Study the drawing (mm; zero at the part's minimum x, y, z) and answer. A direction names the side the tool comes from. Coordinates: 2 decimals unless noted, no trailing zeros. Write each loop counter-clockwise with the first axis right and the second up, starting at its lowest first coordinate (ties: lowest second). Pieces come first, ordered by that corner, then holes. Notation, with made-up numbers: M -14.75,-29.5 L -6.75,-29.5 A19 cw -6.75,1.5 Z; hole C 59,31 d8. An arc over 180 degrees is marked long. Answer as CSV lines item,"result". Start each with the question number.
(1) A cutting plane is placed at B-B on x = 3. Give the vertices of the cut face in (y, z).
(2) A cutting plane is placed at D-D on z = 0.5. Give the vertices of the cut face in (x, y).
(3) Find the intervals of material crossed by L1, parallel to Z at x = 3, y = 0.8; L2, parallel to X at y = 0.5, z = 4; L3, parallel to Y at x = 2.5, z = 0.85, in increasing order. Write a range as [from, to].
(4) For the marked faces 5, 6 and 7, determine the directions among +Z, -Z, +X, -X, +Y, -Y from which every point of the face is accessible in a straight line to the end or side of a thin tool.
(5) Flat-ended cylindrical pins translate along their axes: P1, Ø1.8, axis at x = 3, z = 2.5, coming from the +Y side; P2, Ø2, axis at x = 18, z = 5, coming from the -Y side. Find the tip coordinate at first contact, or state that the pin passes through.
(6) The mould has two halves that part along X. Classify the marked faces 1, 2, 3 and 4: released by +X, released by -X, zero draft, split by the parting line, or undercut.
(7) A cutting plane is placed at C-C on y = 4.5. Give the vertices of the cut face in (x, z), then the cut area to 3 significant figures.
(8) A cutting plane is placed at A-A on z = 4.2. Give the vertices of the cut face in (x, y), then the cut area to 3 significant figures.
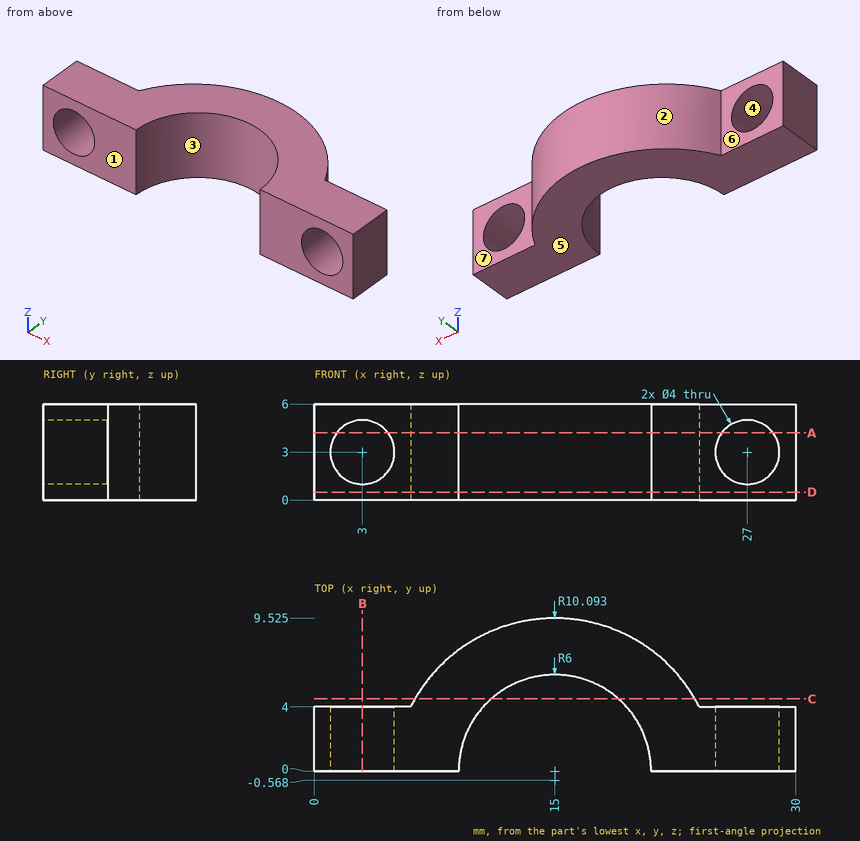
Here are the results:
1,outline,"M 0,0 L 4,0 L 4,1 L 0,1 Z; M 0,5 L 4,5 L 4,6 L 0,6 Z"
2,outline,"M 0,0 L 9,0 A6 cw 21,0 L 30,0 L 30,4 L 24,4 A10.09 ccw 6,4 L 0,4 Z"
3,L1,"z = [0, 1], [5, 6]"
3,L2,"x = [0, 1.27], [4.73, 9.02], [20.98, 25.27], [28.73, 30]"
3,L3,"y = [0, 4]"
4,face 5,"-Z, +X, -X, +Y, -Y"
4,face 6,"+Z, -Z, -X, +Y"
4,face 7,"+Z, -Z, +X, +Y"
5,P1,"passes through"
5,P2,"stops at y = 4.47"
6,face 1,"zero draft"
6,face 2,"split by the parting line"
6,face 3,"undercut"
6,face 4,"undercut"
7,outline,"M 6.27,0 L 11.03,0 L 11.03,6 L 6.27,6 Z; M 18.97,0 L 23.73,0 L 23.73,6 L 18.97,6 Z"
7,area,"57.1 mm^2"
8,outline,"M 0,0 L 1.4,0 L 1.4,4 L 0,4 Z; M 4.6,0 L 9,0 A6 cw 21,0 L 25.4,0 L 25.4,4 L 24,4 A10.09 ccw 6,4 L 4.6,4 Z; M 28.6,0 L 30,0 L 30,4 L 28.6,4 Z"
8,area,"109 mm^2"
